Check sheet for the modelled part. Datum: model origin and axes. Units: mm. A direction names the side the tool comes from. Give positions to 0.01 mm unless a question says otherwise; leave off trailing zeros. Order: outer loops, then holes, each group sorted by start corner. A loop starts at its lowest first (then second) coordinate and runs counter-clockwise, first axis right, second up.
```python
from build123d import *

# Parameters (mm, degrees)
BOSS_EXTRUDE1_DEPTH = 5
SKETCH2_R           = 4.5
CUT_EXTRUDE1_DEPTH  = 6
CUT_EXTRUDE2_DEPTH  = 25
CUT_EXTRUDE3_DEPTH  = 25
FILLET1_R           = 25
SCALE1_SCALE        = 0.225
CUT_EXTRUDE4_REACH  = 3.125
SKETCH5_R           = 1.55
SKETCH7_R           = 1.55
BOSS_EXTRUDE3_DEPTH = 2.26


with BuildPart() as part:
    # Sketch1 → Boss-Extrude1 (new body)
    with BuildSketch(Plane(origin=(0, 0, 0), x_dir=(1, 0, 0), z_dir=(0, 1, 0))):
        with BuildLine():
            ThreePointArc((-130, 0), (-129.975663124, -2.515351975), (-129.902661607, -5.029762169))
            ThreePointArc((-129.902661607, -5.029762169), (-139.064924602, -16.153846154), (-127.596676804, -24.881480435))
            ThreePointArc((-127.596676804, -24.881480435), (-105.812439614, -75.523027104), (-65, -112.583302492))
            ThreePointArc((-65, -112.583302492), (-17.416697508, -65), (0, 0))
            ThreePointArc((0, 0), (-65, -17.416697508), (-130, 0))
        make_face()
    extrude(amount=BOSS_EXTRUDE1_DEPTH)

    # Sketch2 → Cut-Extrude1 (cut, through all)
    with BuildSketch(Plane(origin=(0, 5, 0), x_dir=(1, 0, 0), z_dir=(0, 1, 0))):
        with Locations((-129.131715701, -15)):
            Circle(SKETCH2_R)
        with Locations((-104.833820993, -68.079879377)):
            Circle(SKETCH2_R)
    extrude(amount=-CUT_EXTRUDE1_DEPTH, mode=Mode.SUBTRACT)

    # Sketch3 → Cut-Extrude2 (cut)
    with BuildSketch(Plane(origin=(0, 5, 0), x_dir=(1, 0, 0), z_dir=(0, 1, 0))):
        with BuildLine():
            Line((-34.313010289, -88), (-95.686989711, -88))
            ThreePointArc((-95.686989711, -88), (-81.278298801, -101.458553824), (-65, -112.583302492))
            ThreePointArc((-65, -112.583302492), (-48.721701199, -101.458553824), (-34.313010289, -88))
        make_face()
    extrude(amount=-CUT_EXTRUDE2_DEPTH, mode=Mode.SUBTRACT)

    # Sketch4 → Cut-Extrude3 (cut)
    with BuildSketch(Plane(origin=(0, 5, 0), x_dir=(1, 0, 0), z_dir=(0, 1, 0))):
        with BuildLine():
            ThreePointArc((-130, 0), (-129.975663124, -2.515351975), (-129.902661607, -5.029762169))
            ThreePointArc((-129.902661607, -5.029762169), (-122.310091762, -5.339865772), (-115.00045201, -7.416509169))
            ThreePointArc((-115.00045201, -7.416509169), (-122.619676697, -3.949838105), (-130, 0))
        make_face()
    extrude(amount=-CUT_EXTRUDE3_DEPTH, mode=Mode.SUBTRACT)

    # Fillet1
    fillet1_edges = [part.edges().sort_by_distance(p)[0] for p in [
        (-95.686989711, 2.5, 88),
        (-34.313010289, 2.5, 88),
    ]]
    fillet(fillet1_edges, radius=FILLET1_R)


with BuildPart() as part_1:
    # Scale1: scaled about (-65.342168123, 2.5, 45.115535207)
    add(part.part.scale(SCALE1_SCALE).moved(Location((-50.640180295, 1.9375, 34.964539785))))

    # Sketch5 → Cut-Extrude4 (cut, up to next)
    with BuildSketch(Plane(origin=(0, 3.0625, 0), x_dir=(1, 0, 0), z_dir=(0, 1, 0)), mode=Mode.PRIVATE) as cut_extrude4_sk1:
        with Locations((-79.694816328, -38.339539786)):
            Circle(SKETCH5_R)
    cut_extrude4_tool1 = extrude(cut_extrude4_sk1.sketch, amount=-CUT_EXTRUDE4_REACH, mode=Mode.PRIVATE) & part_1.part
    add(cut_extrude4_tool1.solids().sort_by_distance((-79.694816, 3.0625, 38.33954))[0], mode=Mode.SUBTRACT)

    # Sketch7 → Boss-Extrude3 (add)
    with BuildSketch(Plane.XZ.offset(-1.9375)):
        with Locations((-74.227790019, 50.282512645)):
            Circle(SKETCH7_R)
    extrude(amount=-BOSS_EXTRUDE3_DEPTH)


solid = part_1.part
```
(1) Cross-section at A-A on x = -79. Enter the section's corners in (y, z).
Response values:
outline: (1.94, 36.08) - (3.06, 36.08) - (3.06, 36.95) - (1.94, 36.95) - close; (1.94, 39.73) - (3.06, 39.73) - (3.06, 42.13) - (1.94, 42.13) - close
(2) Cross-section at C-C on z = 38. Enter the section's corners in (x, y).
Response values:
outline: (-81.92, 1.94) - (-81.21, 1.94) - (-81.21, 3.06) - (-81.92, 3.06) - close; (-78.18, 1.94) - (-72.4, 1.94) - (-72.4, 3.06) - (-78.18, 3.06) - close; (-58.13, 1.94) - (-50.8, 1.94) - (-50.8, 3.06) - (-58.13, 3.06) - close
(3) Cross-section at B-B on y = 2.7. Enter the section's corners in (x, z) (3 decimals), then the cut area to 3 significant figures.
Response values:
outline: (-79.868, 36.096) arc R7.262 ccw to (-76.515, 36.633) arc R29.25 cw to (-50.64, 34.965) arc R29.25 ccw to (-56.49, 52.515) arc R5.625 ccw to (-60.99, 54.765) - (-69.54, 54.765) arc R5.625 ccw to (-74.04, 52.515) arc R29.25 ccw to (-74.562, 51.796) arc R1.55 ccw to (-75.746, 49.972) arc R29.25 ccw to (-79.349, 40.563) arc R2.25 ccw (long way) to start; hole circle Ø3.1 at (-79.695, 38.34)
area: 404 mm2
(4) Set-up check for faces 4 (the face through (-75.37, 3.55, 51.33)), 5 (the face through (-78.184, 2.508, 36.162)): record each of +Z, -Z, +X, -X, +Y, -Y from which the full face is reachable in a straight line by a thin tool's end or side.
Response values:
face 4: +Y
face 5: -Z, +Y, -Y
(5) Cross-section at D-D on x = -75. Enter the section's corners in (y, z), then the cut area to 3 significant figures.
Response values:
outline: (1.94, 37.22) - (3.06, 37.22) - (3.06, 48.94) - (4.2, 48.94) - (4.2, 51.63) - (1.94, 51.63) - close
area: 19.3 mm2
(6) Release check for a two-part mould opening along X. For faces 1 (the face through (-67, 3.062, 45)), 2 (the face through (-72.088, 2.492, 54.154)), 3 (the face through (-63.2, 2.49, 38.81)) record: released by +X, released by -X, zero draft, split by the parting line, or undercut.
Response values:
face 1: zero draft
face 2: released by -X
face 3: undercut
(7) Gauge pin test, flat end, axial feed: pin 1 Ø4 at (x, z) = (-76, 41) entering from +Y. Record the tip position at first contact, or that the pin passes through.
Response values:
pin 1: stops at y = 3.06
(8) Material ranges on L1, parallel to Y at x = -75, z = 46.25; L2, parallel to Z at x = -80.5, y = 2.2; L3, parallel to Z at x = -79.5, y = 2.5, recorded low to high.
Response values:
L1: y = 1.94 to 3.06
L2: z = 36.24 to 37.02, 39.66 to 40.44
L3: z = 36.08 to 36.8, 39.88 to 40.58
